Design review of the part built by this model. Coordinates are the model's own, in mm. A direction names the side the tool comes from. Coordinates: 2 decimals unless noted, no trailing zeros. Loops run counter-clockwise (first coordinate to the right, second up) from the corner with the lowest first, then second, coordinate; pieces in that order, holes last. Notation, with made-up numbers: M -1,40 L 22,40 A21 ccw 22,62 Z; hole C -14,67.5 d8. An arc over 180 degrees is marked long. Put each result on its own line as item: value. Start each with the question number.
(1) Clearance check with flat-ended pins moving along their axes: pin 1 (10 mm diameter, centred on y = 102, z = 48, fed in from -X); pin 2 (12 mm diameter, centred on x = -164.5, z = 61.5, fed in from +Y); pin 3 (3 mm diameter, centred on x = -43, z = 65, fed in from +Y). State where each tip first meets the part, or that it passes through.
(2) For probe 1 along X at (y, z) = (50, 40); probe 2 along X at (y, z) = (50, 33); probe 3 along X at (y, z) = (10, 68), list the stretches that pass through material, from the lowest coordinate up. Write a range as [from, to].
(3) The part is to be moulded in two halves that separate along Y. For faces 1 (the cylindrical face through (-117.492, 6.911, 29.551)), 2 (the cylindrical face through (-50, 55, 48)), 3 (the flat face through (-169, 54, 26)), say which applies: +Y half, -Y half, draft (parallel to the pull), parting line (faces both ways), or undercut.
(4) Take a section at B-B, the plane y = 112.5. Give the boundary of the cut face in (x, z), then the cut area to 3 significant figures.
(5) Take a section at A-A, the plane y = 73. Give the boundary of the cut face in (x, z), then the cut area to 3 significant figures.
(6) Take a section at C-C, the plane x = -182. Give the boundary of the cut face in (y, z).
(7) For faces 4 (the cylindrical face through (-83.05, 45.04, 64.33)), 5 (the cylindrical face through (-83.05, 45.04, 32.17)), 6 (the flat face through (-247, 45, 49)), list the 3-axis set-ups (+Z, -Z, +X, -X, +Y, -Y) from which the entire face can be reached by the end or side of a thin tool; tool diameter is ignored.
(8) Take a section at D-D, the plane x = -73. Give the boundary of the cut face in (y, z), then the cut area to 3 significant figures.
```python
from build123d import *

# Parameters (mm, degrees)
SKETCH1_W           = 257
SKETCH1_H           = 96.5
BOSS_EXTRUDE1_DEPTH = 133.5
SKETCH2_W           = 140
SKETCH2_H           = 96.5
CUT_EXTRUDE1_DEPTH  = 45.5
SKETCH3_W           = 52
SKETCH3_H           = 45.75
CUT_EXTRUDE2_DEPTH  = 68
SKETCH4_W           = 68
SKETCH4_H           = 76.5
CUT_EXTRUDE3_DEPTH  = 89
SKETCH5_R           = 5
CUT_EXTRUDE4_DEPTH  = 45.75
SKETCH6_R           = 5
CUT_EXTRUDE5_DEPTH  = 45.75
SKETCH7_R           = 5
CUT_EXTRUDE6_DEPTH  = 97.5
CUT_EXTRUDE7_DEPTH  = 97.5
CUT_EXTRUDE8_DEPTH  = 97.5
SKETCH10_R          = 5
CUT_EXTRUDE9_DEPTH  = 45.75
CUT_EXTRUDE10_DEPTH = 45.75
SKETCH12_R          = 5
CUT_EXTRUDE11_DEPTH = 97.5
SKETCH13_W          = 40
SKETCH13_H          = 28.25
CUT_EXTRUDE12_DEPTH = 134.5
SKETCH14_W          = 20
SKETCH14_H          = 20
CUT_EXTRUDE13_DEPTH = 134.5
CUT_EXTRUDE14_DEPTH = 89
FILLET1_R           = 10
FILLET2_R           = 10


with BuildPart() as part:
    # Sketch1 → Boss-Extrude1 (new body)
    with BuildSketch(Plane(origin=(0, 0, 0), x_dir=(1, 0, 0), z_dir=(0, 1, 0))):
        with Locations((-128.5, -48.25)):
            Rectangle(SKETCH1_W, SKETCH1_H)
    extrude(amount=BOSS_EXTRUDE1_DEPTH)

    # Sketch2 → Cut-Extrude1 (cut)
    with BuildSketch(Plane(origin=(0, 133.5, 0), x_dir=(1, 0, 0), z_dir=(0, 1, 0))):
        with Locations((-187, -48.25)):
            Rectangle(SKETCH2_W, SKETCH2_H)
    extrude(amount=-CUT_EXTRUDE1_DEPTH, mode=Mode.SUBTRACT)

    # Sketch3 → Cut-Extrude2 (cut)
    with BuildSketch(Plane(origin=(0, 88, 0), x_dir=(1, 0, 0), z_dir=(0, 1, 0))):
        with Locations((-143, -22.875)):
            Rectangle(SKETCH3_W, SKETCH3_H)
        with Locations((-143, -73.625)):
            Rectangle(SKETCH3_W, SKETCH3_H)
    extrude(amount=-CUT_EXTRUDE2_DEPTH, mode=Mode.SUBTRACT)

    # Sketch4 → Cut-Extrude3 (cut, through all)
    with BuildSketch(Plane(origin=(0, 88, 0), x_dir=(1, 0, 0), z_dir=(0, 1, 0))):
        with Locations((-213, -48.25)):
            Rectangle(SKETCH4_W, SKETCH4_H)
    extrude(amount=-CUT_EXTRUDE3_DEPTH, mode=Mode.SUBTRACT)

    # Sketch5 → Cut-Extrude4 (cut)
    with BuildSketch(Plane.XY.offset(96.5)):
        with Locations((-154, 10)):
            Circle(SKETCH5_R)
        with BuildLine():
            Line((-169, 20), (-154, 20))
            ThreePointArc((-154, 20), (-146.928932188, 17.071067812), (-144, 10))
            Line((-144, 10), (-144, 6))
            Line((-144, 6), (-117, 6))
            Line((-117, 6), (-117, 88))
            Line((-117, 88), (-169, 88))
            Line((-169, 88), (-169, 20))
        make_face()
    extrude(amount=-CUT_EXTRUDE4_DEPTH, mode=Mode.SUBTRACT)

    # Sketch6 → Cut-Extrude5 (cut)
    with BuildSketch(Plane(origin=(0, 0, 0), x_dir=(-1, 0, 0), z_dir=(0, 0, -1))):
        with Locations((154, 10)):
            Circle(SKETCH6_R)
        with BuildLine():
            Line((144, 6), (117, 6))
            Line((117, 6), (117, 88))
            Line((117, 88), (169, 88))
            Line((169, 88), (169, 20))
            Line((169, 20), (154, 20))
            ThreePointArc((154, 20), (146.928932188, 17.071067812), (144, 10))
            Line((144, 10), (144, 6))
        make_face()
    extrude(amount=-CUT_EXTRUDE5_DEPTH, mode=Mode.SUBTRACT)

    # Sketch7 → Cut-Extrude6 (cut, through all)
    with BuildSketch(Plane(origin=(0, 0, 0), x_dir=(-1, 0, 0), z_dir=(0, 0, -1))):
        with Locations((154, 10)):
            Circle(SKETCH7_R)
    extrude(amount=-CUT_EXTRUDE6_DEPTH, mode=Mode.SUBTRACT)

    # Sketch8 → Cut-Extrude7 (cut, through all)
    with BuildSketch(Plane.XY.offset(96.5)):
        Polygon((0, 40), (-80.638168804, 40), (-114.202154051, 0), (0, 0), align=None)
    extrude(amount=-CUT_EXTRUDE7_DEPTH, mode=Mode.SUBTRACT)

    # Sketch9 → Cut-Extrude8 (cut, through all)
    with BuildSketch(Plane.XY.offset(96.5)):
        Polygon((-65.168254999, 133.5), (-103.347288218, 88), (-117, 88), (-117, 133.5), align=None)
    extrude(amount=-CUT_EXTRUDE8_DEPTH, mode=Mode.SUBTRACT)

    # Sketch10 → Cut-Extrude9 (cut)
    with BuildSketch(Plane.XY.offset(96.5)):
        with Locations((-50, 50)):
            Circle(SKETCH10_R)
        with BuildLine():
            Line((-83.436014753, 46), (-60, 46))
            Line((-60, 46), (-60, 50))
            ThreePointArc((-60, 50), (-57.071067812, 57.071067812), (-50, 60))
            Line((-50, 60), (-40, 60))
            Line((-40, 60), (-40, 133.5))
            Line((-40, 133.5), (-65.168254999, 133.5))
            Line((-65.168254999, 133.5), (-103.347288218, 88))
            Line((-103.347288218, 88), (-117, 88))
            Line((-117, 88), (-117, 6))
            Line((-117, 6), (-83.436014753, 46))
        make_face()
    extrude(amount=-CUT_EXTRUDE9_DEPTH, mode=Mode.SUBTRACT)

    # Sketch11 → Cut-Extrude10 (cut)
    with BuildSketch(Plane(origin=(0, 0, 0), x_dir=(-1, 0, 0), z_dir=(0, 0, -1))):
        with BuildLine():
            Line((65.168254999, 133.5), (40, 133.5))
            Line((40, 133.5), (40, 60))
            Line((40, 60), (50, 60))
            ThreePointArc((50, 60), (57.071067812, 57.071067812), (60, 50))
            Line((60, 50), (60, 46))
            Line((60, 46), (83.436014753, 46))
            Line((83.436014753, 46), (117, 6))
            Line((117, 6), (117, 88))
            Line((117, 88), (103.347288218, 88))
            Line((103.347288218, 88), (65.168254999, 133.5))
        make_face()
    extrude(amount=-CUT_EXTRUDE10_DEPTH, mode=Mode.SUBTRACT)

    # Sketch12 → Cut-Extrude11 (cut, through all)
    with BuildSketch(Plane(origin=(0, 0, 0), x_dir=(-1, 0, 0), z_dir=(0, 0, -1))):
        with Locations((50, 50)):
            Circle(SKETCH12_R)
    extrude(amount=-CUT_EXTRUDE11_DEPTH, mode=Mode.SUBTRACT)

    # Sketch13 → Cut-Extrude12 (cut, through all)
    with BuildSketch(Plane(origin=(0, 133.5, 0), x_dir=(1, 0, 0), z_dir=(0, 1, 0))):
        with Locations((-20, -82.375)):
            Rectangle(SKETCH13_W, SKETCH13_H)
        with Locations((-20, -14.125)):
            Rectangle(SKETCH13_W, SKETCH13_H)
    extrude(amount=-CUT_EXTRUDE12_DEPTH, mode=Mode.SUBTRACT)

    # Sketch14 → Cut-Extrude13 (cut, through all)
    with BuildSketch(Plane(origin=(0, 133.5, 0), x_dir=(1, 0, 0), z_dir=(0, 1, 0))):
        with Locations((-20, -48.25)):
            Rectangle(SKETCH14_W, SKETCH14_H)
    extrude(amount=-CUT_EXTRUDE13_DEPTH, mode=Mode.SUBTRACT)

    # Sketch15 → Cut-Extrude14 (cut, through all)
    with BuildSketch(Plane(origin=(0, 88, 0), x_dir=(1, 0, 0), z_dir=(0, 1, 0))):
        Polygon((-207, 0), (-20, -28.25), (-20, 0), align=None)
        Polygon((-207, -96.5), (-20, -68.25), (-20, -96.5), align=None)
    extrude(amount=-CUT_EXTRUDE14_DEPTH, mode=Mode.SUBTRACT)

    # Fillet1
    fillet1_edges = [part.edges().sort_by_distance(p)[0] for p in [
        (-117, 6, 29.673128342),
        (-83.436014753, 46, 64.291624109),
        (-65.168254999, 133.5, 48.25),
        (-103.347288218, 88, 48.25),
        (-83.436014753, 46, 32.208375891),
        (-114.202154051, 0, 48.25),
        (-117, 6, 66.826871658),
    ]]
    fillet(fillet1_edges, radius=FILLET1_R)

    # Fillet2
    fillet2_edges = [part.edges().sort_by_distance(p)[0] for p in [
        (-80.638168804, 40, 48.25),
    ]]
    fillet(fillet2_edges, radius=FILLET2_R)


solid = part.part
```
Computed values:
1. pin 1: stops at x = -95.8
1. pin 2: stops at y = 88
1. pin 3: stops at y = 60
2. probe 1: x = [-257, -247], [-179, -169], [-60, -55], [-45, -30], [-10, 0]
2. probe 2: x = [-257, -247], [-179, -169], [-60, -55], [-45, 0]
2. probe 3: x = [-257, -247], [-179, -159], [-149, -144], [-113.64, -105.81]
3. face 1: +Y half
3. face 2: undercut
3. face 3: draft
4. outline: M -82.79,45.75 L -40,45.75 L -40,28.25 L 0,28.25 L 0,68.25 L -40,68.25 L -40,50.75 L -82.79,50.75 Z; hole M -30,38.25 L -10,38.25 L -10,58.25 L -30,58.25 Z
4. area: 1,410 mm^2
5. outline: M -257,0 L -207,0 L -169,5.74 L -169,45.75 L -40,45.75 L -40,28.25 L 0,28.25 L 0,68.25 L -40,68.25 L -40,50.75 L -169,50.75 L -169,90.76 L -207,96.5 L -257,96.5 Z; hole M -247,10 L -179,10 L -179,86.5 L -247,86.5 Z; hole M -30,38.25 L -10,38.25 L -10,58.25 L -30,58.25 Z
5. area: 4,920 mm^2
6. outline: M 0,3.78 L 88,3.78 L 88,10 L 0,10 Z; M 0,86.5 L 88,86.5 L 88,92.72 L 0,92.72 Z
7. face 4: +Z, +Y
7. face 5: -Z, +Y
7. face 6: +Y, -Y
8. outline: M 40,20.24 L 46,20.24 L 46,45.75 L 124.17,45.75 L 124.17,50.75 L 46,50.75 L 46,76.26 L 40,76.26 Z
8. area: 727 mm^2
